CAD build for the part. Positions are in the model's coordinates, mm. A direction names the side the tool comes from. Give positions to 0.01 mm unless a question says otherwise; leave off trailing zeros. Write each loop counter-clockwise with the first axis right and the second up, starting at its lowest first coordinate (ties: lowest second). Pieces come first, ordered by that corner, then holes. Notation, with made-up numbers: (37.5, 6) -> (42.5, 6) arc R15 ccw to (42.5, 18) -> close; hole circle Ø9 at (74.5, -13.75). An arc over 180 degrees is marked (long way). Answer as a JSON object with one key per item and string values.
```python
from build123d import *
from build123d.topology import SkipClean

# Parameters (mm, degrees)
SKETCH1_R           = 9.95
SKETCH1_R_2         = 4.5
SKETCH1_R_3         = 1.6
BOSS_EXTRUDE1_DEPTH = 7
BOSS_EXTRUDE3_START = 0.5
SKETCH3_R           = 4.5
BOSS_EXTRUDE3_DEPTH = 0.5
BOSS_EXTRUDE4_START = 3
SKETCH5_R           = 3
SKETCH5_R_2         = 4.5
BOSS_EXTRUDE4_DEPTH = 3
SKETCH6_R           = 4.05
BOSS_EXTRUDE5_DEPTH = 1.5
BOSS_EXTRUDE6_START = 3
SKETCH7_R           = 3.25
BOSS_EXTRUDE6_DEPTH = 3
CHAMFER1_SIZE       = 0.8
CUT_EXTRUDE1_START  = -1
CUT_EXTRUDE1_DEPTH  = 1
SKETCH9_R           = 1.6
CUT_EXTRUDE2_DEPTH  = 37.724772234
BOSS_EXTRUDE7_DEPTH = 2
CUT_EXTRUDE3_DEPTH  = 2
CUT_EXTRUDE3_DRAFT  = -5


with BuildPart() as part:
    # Sketch1 → Boss-Extrude1 (new body)
    with BuildSketch(Plane.XY):
        Circle(SKETCH1_R)
        Circle(SKETCH1_R_2, mode=Mode.SUBTRACT)
        with Locations((-5.656854249, -5.656854249)):
            Circle(SKETCH1_R_3, mode=Mode.SUBTRACT)
        with Locations((-5.656854249, 5.656854249)):
            Circle(SKETCH1_R_3, mode=Mode.SUBTRACT)
        with Locations((5.656854249, 5.656854249)):
            Circle(SKETCH1_R_3, mode=Mode.SUBTRACT)
        with Locations((5.656854249, -5.656854249)):
            Circle(SKETCH1_R_3, mode=Mode.SUBTRACT)
    extrude(amount=-BOSS_EXTRUDE1_DEPTH)

    # Sketch3 → Boss-Extrude3 (add)
    # profile 1 of 5: a face of its own
    with BuildSketch(Plane.XY.offset(BOSS_EXTRUDE3_START)):
        with BuildLine():
            ThreePointArc((4.586976758, 8.829617445), (0, 9.95), (-4.586976758, 8.829617445))
            Line((-4.586976758, 8.829617445), (-3.535533906, 7.778174593))
            ThreePointArc((-3.535533906, 7.778174593), (-3.535533906, 3.535533906), (-7.778174593, 3.535533906))
            Line((-7.778174593, 3.535533906), (-8.829617445, 4.586976758))
            ThreePointArc((-8.829617445, 4.586976758), (-9.95, 0), (-8.829617445, -4.586976758))
            Line((-8.829617445, -4.586976758), (-7.778174593, -3.535533906))
            ThreePointArc((-7.778174593, -3.535533906), (-3.535533906, -3.535533906), (-3.535533906, -7.778174593))
            Line((-3.535533906, -7.778174593), (-4.586976758, -8.829617445))
            ThreePointArc((-4.586976758, -8.829617445), (0, -9.95), (4.586976758, -8.829617445))
            Line((4.586976758, -8.829617445), (3.535533906, -7.778174593))
            ThreePointArc((3.535533906, -7.778174593), (3.535533906, -3.535533906), (7.778174593, -3.535533906))
            Line((7.778174593, -3.535533906), (8.829617445, -4.586976758))
            ThreePointArc((8.829617445, -4.586976758), (9.665846926, -2.360911521), (9.95, 0))
            ThreePointArc((9.95, 0), (9.665846926, 2.360911521), (8.829617445, 4.586976758))
            Line((8.829617445, 4.586976758), (7.778174593, 3.535533906))
            ThreePointArc((7.778174593, 3.535533906), (3.535533906, 3.535533906), (3.535533906, 7.778174593))
            Line((3.535533906, 7.778174593), (4.586976758, 8.829617445))
        make_face()
        Circle(SKETCH3_R, mode=Mode.SUBTRACT)
    # profile 2 of 5: a face of its own
    with BuildSketch(Plane.XY.offset(BOSS_EXTRUDE3_START)):
        with BuildLine():
            Line((-8.829617445, 4.586976758), (-9.420721004, 5.178080317))
            ThreePointArc((-9.420721004, 5.178080317), (-10.75, 0), (-9.420721004, -5.178080317))
            Line((-9.420721004, -5.178080317), (-8.829617445, -4.586976758))
            ThreePointArc((-8.829617445, -4.586976758), (-9.95, 0), (-8.829617445, 4.586976758))
        make_face()
    # profile 3 of 5: a face of its own
    with BuildSketch(Plane.XY.offset(BOSS_EXTRUDE3_START)):
        with BuildLine():
            ThreePointArc((5.178080317, 9.420721004), (0, 10.75), (-5.178080317, 9.420721004))
            Line((-5.178080317, 9.420721004), (-4.586976758, 8.829617445))
            ThreePointArc((-4.586976758, 8.829617445), (0, 9.95), (4.586976758, 8.829617445))
            Line((4.586976758, 8.829617445), (5.178080317, 9.420721004))
        make_face()
    # profile 4 of 5: a face of its own
    with BuildSketch(Plane.XY.offset(BOSS_EXTRUDE3_START)):
        with BuildLine():
            ThreePointArc((10.75, 0), (10.41237847, 2.672989825), (9.420721004, 5.178080317))
            Line((9.420721004, 5.178080317), (8.829617445, 4.586976758))
            ThreePointArc((8.829617445, 4.586976758), (9.665846926, 2.360911521), (9.95, 0))
            ThreePointArc((9.95, 0), (9.665846926, -2.360911521), (8.829617445, -4.586976758))
            Line((8.829617445, -4.586976758), (9.420721004, -5.178080317))
            ThreePointArc((9.420721004, -5.178080317), (10.41237847, -2.672989825), (10.75, 0))
        make_face()
    # profile 5 of 5: a face of its own
    with BuildSketch(Plane.XY.offset(BOSS_EXTRUDE3_START)):
        with BuildLine():
            Line((-4.586976758, -8.829617445), (-5.178080317, -9.420721004))
            ThreePointArc((-5.178080317, -9.420721004), (0, -10.75), (5.178080317, -9.420721004))
            Line((5.178080317, -9.420721004), (4.586976758, -8.829617445))
            ThreePointArc((4.586976758, -8.829617445), (0, -9.95), (-4.586976758, -8.829617445))
        make_face()
    extrude(amount=-BOSS_EXTRUDE3_DEPTH)

    # Sketch5 → Boss-Extrude4 (add)
    with SkipClean():  # the faces are left unmerged after this step: merging them gives an invalid solid
        with BuildSketch(Plane.XY.offset(0.5).offset(BOSS_EXTRUDE4_START)):
            with BuildLine():
                Line((-5.178080317, 9.420721004), (19.562128784, 24.012569881))
                ThreePointArc((19.562128784, 24.012569881), (23.511300474, 23.511300474), (24.012569881, 19.562128784))
                Line((24.012569881, 19.562128784), (9.420721004, -5.178080317))
                Line((9.420721004, -5.178080317), (7.778174593, -3.535533906))
                ThreePointArc((7.778174593, -3.535533906), (3.535533906, -3.535533906), (3.535533906, -7.778174593))
                Line((3.535533906, -7.778174593), (5.178080317, -9.420721004))
                ThreePointArc((5.178080317, -9.420721004), (0, -10.75), (-5.178080317, -9.420721004))
                Line((-5.178080317, -9.420721004), (-3.535533906, -7.778174593))
                ThreePointArc((-3.535533906, -7.778174593), (-3.535533906, -3.535533906), (-7.778174593, -3.535533906))
                Line((-7.778174593, -3.535533906), (-9.420721004, -5.178080317))
                ThreePointArc((-9.420721004, -5.178080317), (-10.75, 0), (-9.420721004, 5.178080317))
                Line((-9.420721004, 5.178080317), (-7.778174593, 3.535533906))
                ThreePointArc((-7.778174593, 3.535533906), (-3.535533906, 3.535533906), (-3.535533906, 7.778174593))
                Line((-3.535533906, 7.778174593), (-5.178080317, 9.420721004))
            make_face()
            with Locations(Location((5.656854249, 5.656854249, 0), (0, 0, 135))):
                Circle(SKETCH5_R, mode=Mode.SUBTRACT)
            Circle(SKETCH5_R_2, mode=Mode.SUBTRACT)
        extrude(amount=-BOSS_EXTRUDE4_DEPTH)

    # Sketch6 → Boss-Extrude5 (add)
    with SkipClean():  # the faces are left unmerged after this step: merging them gives an invalid solid
        with BuildSketch(Plane(origin=(0, 0, 3.5), x_dir=(-1, 0, 0), z_dir=(0, 0, -1))):
            with Locations((-21.213203436, 21.213203436)):
                Circle(SKETCH6_R)
        extrude(amount=-BOSS_EXTRUDE5_DEPTH)

    # Sketch7 → Boss-Extrude6 (add)
    with SkipClean():  # the faces are left unmerged after this step: merging them gives an invalid solid
        with BuildSketch(Plane.XY.offset(5).offset(BOSS_EXTRUDE6_START)):
            with Locations((21.213203436, 21.213203436)):
                Circle(SKETCH7_R)
        extrude(amount=-BOSS_EXTRUDE6_DEPTH)

    # Chamfer1
    # the kernel refuses this chamfer: 0.8 mm, written as the material it adds along each edge
    with BuildSketch(Plane(origin=(24.012569881, 19.562128784, 3.5), x_dir=(-0.02368339518990366, 0.013968536890575577, -0.9996219169112968), z_dir=(-0.5080229697131419, -0.8613435216241195, 0))) as chamfer1_piece_1_section:
        Polygon((CHAMFER1_SIZE * 0.999621916911, CHAMFER1_SIZE * 0.0274958766106), (-CHAMFER1_SIZE * 0.0274958766106, CHAMFER1_SIZE * 0.999621916911), (0, 0), align=None)
    chamfer1_piece_1 = extrude(amount=4.473955585, mode=Mode.PRIVATE)
    chamfer1_piece_1 = chamfer1_piece_1 & Plane(origin=(21.213203436, 21.213203436, 3.215245779), x_dir=(-1, 0, 0), z_dir=(0, 0, -1)) * Cylinder(4.05, 13, mode=Mode.PRIVATE)
    add(chamfer1_piece_1)
    with BuildSketch(Plane(origin=(21.213203436, 21.213203436, 3.5), x_dir=(-0.508022969713124, 0.8613435216241301, 0), z_dir=(-0.8613435216241301, -0.508022969713124, 0))) as chamfer1_piece_2:
        Polygon((3.25, CHAMFER1_SIZE), (3.25 + CHAMFER1_SIZE, 0), (3.25, 0), align=None)
    revolve(axis=Axis((21.213203436, 21.213203436, 3.5), (0, 0, -1)), revolution_arc=151.064460502)
    with BuildSketch(Plane(origin=(15.708516125, 21.739697678, 3.5), x_dir=(0.01396853689057517, -0.0236833951899039, -0.9996219169112968), z_dir=(0.8613435216241283, 0.508022969713127, 0))) as chamfer1_piece_3_section:
        Polygon((CHAMFER1_SIZE * 0.999621916911, CHAMFER1_SIZE * 0.0274958766106), (-CHAMFER1_SIZE * 0.0274958766106, CHAMFER1_SIZE * 0.999621916911), (0, 0), align=None)
    chamfer1_piece_3 = extrude(amount=4.473955585, mode=Mode.PRIVATE)
    chamfer1_piece_3 = chamfer1_piece_3 & Plane(origin=(21.213203436, 21.213203436, 3.215245779), x_dir=(-1, 0, 0), z_dir=(0, 0, -1)) * Cylinder(4.05, 13, mode=Mode.PRIVATE)
    add(chamfer1_piece_3)

    # Sketch8 → Cut-Extrude1 (cut)
    with BuildSketch(Plane(origin=(0, 0, 0.5), x_dir=(-1, 0, 0), z_dir=(0, 0, -1)).offset(CUT_EXTRUDE1_START)):
        with BuildLine():
            Line((-22.803705141, 18.398307761), (-19.570683125, 18.428340717))
            Line((-19.570683125, 18.428340717), (-17.98018142, 21.243236391))
            Line((-17.98018142, 21.243236391), (-19.62270173, 24.02809911))
            Line((-19.62270173, 24.02809911), (-19.639679475, 24.056884561))
            ThreePointArc((-19.639679475, 24.056884561), (-23.542662563, 23.479504425), (-24.012569881, 19.562128784))
            Line((-24.012569881, 19.562128784), (-23.326144782, 18.398307761))
            Line((-23.326144782, 18.398307761), (-22.803705141, 18.398307761))
        make_face()
    extrude(amount=CUT_EXTRUDE1_DEPTH, mode=Mode.SUBTRACT)

    # Sketch9 → Cut-Extrude2 (cut, through all)
    with BuildSketch(Plane(origin=(0, 0, 1.5), x_dir=(-1, 0, 0), z_dir=(0, 0, -1))):
        with Locations((-21.213203436, 21.213203436)):
            Circle(SKETCH9_R)
    extrude(amount=-CUT_EXTRUDE2_DEPTH, mode=Mode.SUBTRACT)

    # Sketch10 → Boss-Extrude7 (add)
    with BuildSketch(Plane(origin=(0, 0, -7), x_dir=(-1, 0, 0), z_dir=(0, 0, -1))):
        with BuildLine():
            ThreePointArc((9.610301508, 2.577713121), (7.35, 0), (9.610301508, -2.577713121))
            ThreePointArc((9.610301508, -2.577713121), (9.95, 0), (9.610301508, 2.577713121))
        make_face()
    extrude(amount=BOSS_EXTRUDE7_DEPTH)


with BuildPart() as cut_extrude3_tool:
    # Sketch11 → Cut-Extrude3 (with draft: the straight prism first)
    with BuildSketch(Plane(origin=(0, 0, -7), x_dir=(-1, 0, 0), z_dir=(0, 0, -1))):
        with BuildLine():
            ThreePointArc((-2.26467179, -4.332286617), (-3.630697194, -3.966261214), (-3.996722598, -5.332286617))
            Line((-3.996722598, -5.332286617), (-3.246722598, -6.631324723))
            ThreePointArc((-3.246722598, -6.631324723), (-1.880697194, -6.997350127), (-1.51467179, -5.631324723))
            Line((-1.51467179, -5.631324723), (-2.26467179, -4.332286617))
        make_face()
    extrude(amount=-CUT_EXTRUDE3_DEPTH)
    # Cut-Extrude3: the draft: its side faces are tilted about the plane it starts from
    cut_extrude3_sides = [cut_extrude3_tool.faces().sort_by_distance(p)[0] for p in [
        (1.880697194, -6.997350127, -6),
        (1.88967179, -4.98180567, -6),
        (3.630697194, -3.966261214, -6),
        (3.621722598, -5.98180567, -6),
    ]]
    draft(cut_extrude3_sides, Plane(origin=(0, 0, -7), x_dir=(-1, 0, 0), z_dir=(0, 0, -1)), CUT_EXTRUDE3_DRAFT)


with BuildPart() as part_1:
    add(part.part)

    # Cut-Extrude3: cut by cut_extrude3_tool
    add(cut_extrude3_tool.part, mode=Mode.SUBTRACT)


solid = part_1.part
```
1) Mould opens along X. For faces 4 (the flat face through (-0.1, 10.2, 0)), 5 (the flat face through (7.019, 16.615, 2.021)), 6 (the cylindrical face through (-3.58, 3.49, 1.77)) say: released by +X, released by -X, zero draft, split by the parting line, or undercut.
Model answer:
{"face 4": "zero draft", "face 5": "released by -X", "face 6": "undercut"}
2) Slice it at D-D (z = -3.25). List the corners of the cut face in (x, y).
Model answer:
{"outline": "circle Ø19.9 at (0, 0); hole circle Ø3.2 at (-5.66, -5.66); hole circle Ø3.2 at (-5.66, 5.66); hole circle Ø9 at (0, 0); hole circle Ø3.2 at (5.66, -5.66); hole circle Ø3.2 at (5.66, 5.66)"}
3) Slice it at B-B (x = 0). List the corners of the cut face in (y, z), then the cut area to 3 significant figures.
Model answer:
{"outline": "(-10.75, 0) -> (-9.95, 0) -> (-9.95, -7) -> (-4.5, -7) -> (-4.5, 3.5) -> (-10.75, 3.5) -> close; (4.5, -7) -> (9.95, -7) -> (9.95, 0) -> (10.75, 0) -> (10.75, 0.5) -> (12.47, 0.5) -> (12.47, 3.5) -> (4.5, 3.5) -> close", "area": "125 mm2"}
4) Wall check: probe 1 along Y at (x, z) = (-0.5, -2); probe 2 along Y at (x, z) = (2, -6.75); probe 3 along X at (y, z) = (4, -1). Give the ranges that are in metal, low to high.
Model answer:
{"probe 1": "y = -9.94 to -4.47, 4.47 to 9.94", "probe 2": "y = -9.75 to -7.03, -4.83 to -4.03, 4.03 to 9.75", "probe 3": "x = -9.11 to -2.06, 2.06 to 9.11"}
5) Slice it at A-A (z = -5.75). List the corners of the cut face in (x, y).
Model answer:
{"outline": "circle Ø19.9 at (0, 0); hole circle Ø3.2 at (-5.66, -5.66); hole circle Ø3.2 at (-5.66, 5.66); hole circle Ø9 at (0, 0); hole (1.61, -5.69) arc R0.89 ccw to (3.15, -6.58) -> (3.9, -5.28) arc R0.89 ccw to (2.36, -4.39) -> close; hole circle Ø3.2 at (5.66, -5.66); hole circle Ø3.2 at (5.66, 5.66)"}
6) 3-axis set-ups, long thin cutter, end or side, ignore diameter. For faces 1 (the flat face through (-4.37, -8.61, 1.77)), 2 (the cylindrical face through (23.47, 23.55, 2.1)), 3 (the flat face through (4, -4, 0)): which of +Z, -Z, +X, -X, +Y, -Y reach the whole face in a straight line?
Model answer:
{"face 1": "+Z, -X", "face 2": "-Z", "face 3": "+Z"}
7) Pin check, flat tips, straight feed: pin 1 (4 mm diameter, centred on x = 5.66, y = -5.66, fed in from +Z); pin 2 (5 mm diameter, centred on x = 5.5, y = -6.5, fed in from +Z); pin 3 (5 mm diameter, centred on x = -5.66, y = -5.66, fed in from -Z). Stop position of each tip, or through.
Model answer:
{"pin 1": "stops at z = 0", "pin 2": "stops at z = 3.5", "pin 3": "stops at z = -7"}
8) Slice it at C-C (z = 2). List the corners of the cut face in (x, y).
Model answer:
{"outline": "(-9.42, -5.18) -> (-7.78, -3.54) arc R3 cw to (-3.54, -7.78) -> (-5.18, -9.42) arc R10.75 ccw to (5.18, -9.42) -> (3.54, -7.78) arc R3 cw to (7.78, -3.54) -> (9.42, -5.18) -> (24.01, 19.56) arc R3.25 ccw to (19.56, 24.01) -> (-5.18, 9.42) -> (-3.54, 7.78) arc R3 cw to (-7.78, 3.54) -> (-9.42, 5.18) arc R10.75 ccw to start; hole circle Ø9 at (0, 0); hole circle Ø6 at (5.66, 5.66); hole circle Ø3.2 at (21.21, 21.21)"}
